Geometry check sheet. Reference: the model listing, model coordinates, mm. Give positions to 0.01 mm unless a question says otherwise; leave off trailing zeros. Loops run counter-clockwise (first coordinate to the right, second up) from the corner with the lowest first, then second, coordinate; pieces in that order, holes last. Notation, with made-up numbers: (79, -2) -> (135, -2) arc R29 cw to (135, 23) -> close; hole circle Ø1 at (26, 5). An arc over 180 degrees is marked (long way). Write each question's results on one line, items separated by ' | '. Start each with the question number.
1) Sectioned sample at A-A on y = 187. Record the cut outline in (x, z).
2) Sectioned sample at B-B on x = -117. Record the cut outline in (y, z), then the cut area to 3 significant figures.
3) Depth check by flat-ended pin: pin 1 (11 mm diameter, centred on x = -117, y = 187, fed in from +Z); pin 2 (6 mm diameter, centred on x = 118, y = -191.5, fed in from -Z). Enter the tip coordinate at first touch or a pass-through.
4) Scan lines: line 1 (X direction, y = -187, z = 7.25); line 2 (Y direction, x = 117, z = 9.5); line 3 (X direction, y = 187, z = 26.25). Record each from-to range of solid material in increasing order. Write a range as from..to.
Autodesk Inventor part; units mm, degrees
ref_plane "YZ Plane" through (0, 0, 0) normal (1, 0, 0) x (0, 1, 0)
ref_plane "XZ Plane" through (0, 0, 0) normal (0, 1, 0) x (-1, 0, 0)
ref_plane "XY Plane" through (0, 0, 0) normal (0, 0, 1) x (1, 0, 0)
sketch "Sketch1" plane through (0, 0, 0) normal (0, 0, 1) x (1, 0, 0)
  line L0 (-130, 200) -> (130, 200)
  line L1 (130, 200) -> (130, -200)
  line L2 (130, -200) -> (-130, -200)
  line L3 (-130, -200) -> (-130, 200)
  point P0 (0, 0)
  point P1 (-130, 0)
  point P2 (0, 200)
  point P3 (-117, 187)
  dimension "d74" = 117
  dimension "d75" = 187
  dimension "d92" = 260
  dimension "d93" = 400
extrude "Extrusion1" add sketch "Sketch1" along normal blind 30
hole "Hole1" at (-117, 187, 0) direction (0, 0, 1) diameter 14 depth 30 counterbore diameter 20 counterbore depth 13
pattern_linear "Rectangular Pattern1" count 2 spacing 374 along (0, -1, 0) count 2 spacing 234 along (1, 0, 0) of "Hole1"
chamfer "Chamfer1" distance 0.5 angle 45 12 edges at (-130, 0, 30) (-130, -200, 15) (-130, 0, 0) (-130, 200, 15) (0, 200, 30) (0, 200, 0) (130, 200, 15) (130, 0, 0) (130, 0, 30) (0, -200, 30) (0, -200, 0) (130, -200, 15)
equation "\"d92\" = W_"
equation "\"d93\" = L"
equation "\"d20\" = H_"
equation "\"d76\" = S2_d1"
equation "\"d78\" = S2_d2"
equation "\"d79\" = S2_k"
equation "\"d81\" = H_"
equation "\"L\" = 400"
equation "\"W_\" = 260"
equation "\"H_\" = 30"
equation "\"S2_W\" = 234"
equation "\"S2_d1\" = 14"
equation "\"S2_d2\" = 20"
equation "\"S2_k\" = 13"
equation "\"S2_L\" = 374"
properties part number "SA-EP-400x260x30" material "S 55 C"
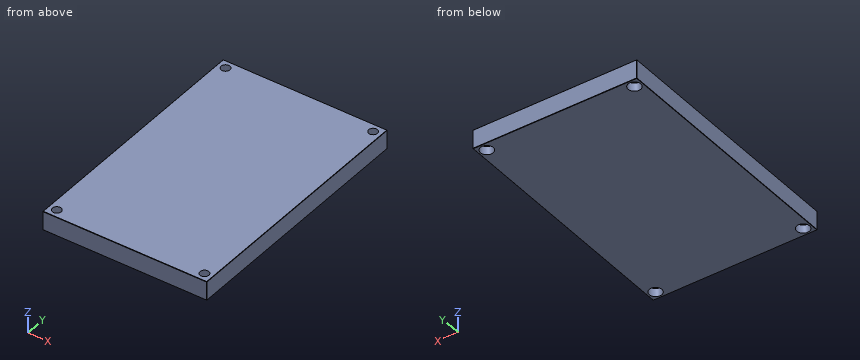
Result:
1) outline: (-130, 0.5) -> (-129.5, 0) -> (-127, 0) -> (-127, 13) -> (-124, 13) -> (-124, 30) -> (-129.5, 30) -> (-130, 29.5) -> close; (-110, 13) -> (-107, 13) -> (-107, 0) -> (107, 0) -> (107, 13) -> (110, 13) -> (110, 30) -> (-110, 30) -> close; (124, 13) -> (127, 13) -> (127, 0) -> (129.5, 0) -> (130, 0.5) -> (130, 29.5) -> (129.5, 30) -> (124, 30) -> close
2) outline: (-200, 0.5) -> (-199.5, 0) -> (-197, 0) -> (-197, 13) -> (-194, 13) -> (-194, 30) -> (-199.5, 30) -> (-200, 29.5) -> close; (-180, 13) -> (-177, 13) -> (-177, 0) -> (177, 0) -> (177, 13) -> (180, 13) -> (180, 30) -> (-180, 30) -> close; (194, 13) -> (197, 13) -> (197, 0) -> (199.5, 0) -> (200, 0.5) -> (200, 29.5) -> (199.5, 30) -> (194, 30) -> close | area: 11,000 mm^2
3) pin 1: through | pin 2: z = 13
4) line 1: -130..-127, -107..107, 127..130 | line 2: -200..-197, -177..177, 197..200 | line 3: -130..-124, -110..110, 124..130
